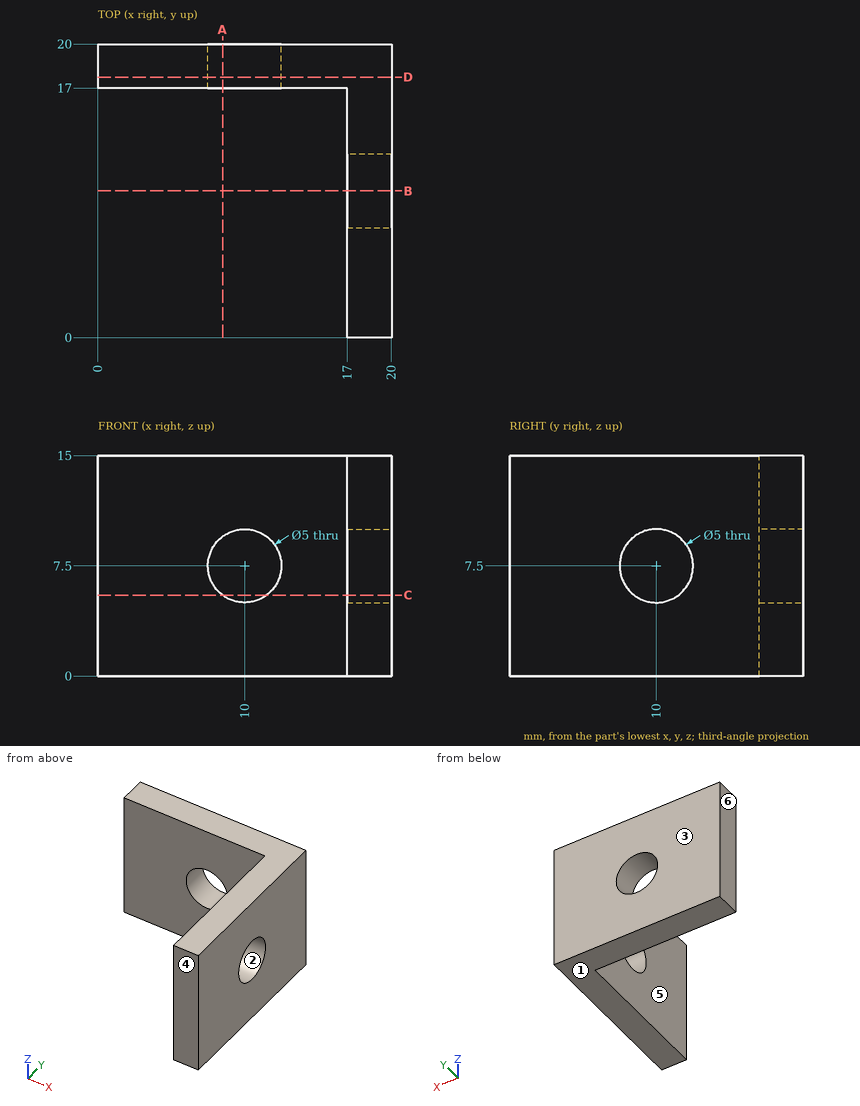
Could you check a few things on this drawing? It's one solid part, dimensions in mm from its lowest x, y, z. A direction names the side the tool comes from. Round coordinates to 2 decimals unless told otherwise and drop trailing zeros. Order: outer loops, then holes, each group sorted by start corner. A loop starts at its lowest first (then second) coordinate and runs counter-clockwise, first axis right, second up. Notation, with made-up numbers: M 76.25,36 L 110.25,36 A36 cw 110.25,75 Z; hole C 36.25,47.5 d3. An arc over 180 degrees is marked long. One line per question, with ' | ' between items. Start each with the question number.
(1) Suppose I cut it at A-A on x = 8.5. List the corners of the cut face in (y, z) for me, then the cut area to 3 significant figures.
(2) Suppose I cut it at B-B on y = 10. List the corners of the cut face in (x, z) for me, then the cut area to 3 significant figures.
(3) Suppose I cut it at C-C on z = 5.5. List the corners of the cut face in (x, y) for me, then the cut area to 3 significant figures.
(4) For P1, Ø5, axis at x = 8.5, y = 14, coming from the +Z side; P2, Ø7.5, axis at x = 11, z = 5, coming from the -Y side; P3, Ø6.5, axis at y = 10, z = 7.5, coming from the -X side, each with a flat end and sliding along its axis, tell me the tip position at first contact or that it passes through.
(5) Thinking about a two-plate mould opening in Y: for the marked faces 1, 2, 3 and 4, which applies, +Y half, -Y half, draft (parallel to the pull), parting line (faces both ways), or undercut?
(6) Suppose I cut it at D-D on y = 17.75. List the corners of the cut face in (x, z) for me.
(7) Please list where these lines run through material, in increasing order: line 1 along X through (y, z) = (17.95, 7.5); line 2 along Z through (x, y) = (19, 10); line 3 along X through (y, z) = (2.5, 6.75).
(8) For the marked faces 5 and 6, which set-ups out of +Z, -Z, +X, -X, +Y, -Y let a thin tool reach every point of the face, with its end or its side?
Geometry results:
1) outline: M 17,0 L 20,0 L 20,5.5 L 17,5.5 Z; M 17,9.5 L 20,9.5 L 20,15 L 17,15 Z | area: 33.0 mm²
2) outline: M 17,0 L 20,0 L 20,5 L 17,5 Z; M 17,10 L 20,10 L 20,15 L 17,15 Z | area: 30.0 mm²
3) outline: M 0,17 L 8.5,17 L 8.5,20 L 0,20 Z; M 11.5,17 L 17,17 L 17,11.5 L 20,11.5 L 20,20 L 11.5,20 Z; M 17,0 L 20,0 L 20,8.5 L 17,8.5 Z | area: 93.0 mm²
4) P1: through | P2: y = 17 | P3: x = 17
5) face 1: draft | face 2: undercut | face 3: +Y half | face 4: -Y half
6) outline: M 0,0 L 20,0 L 20,15 L 0,15 Z; hole C 10,7.5 d5
7) line 1: 0 to 7.5, 12.5 to 20 | line 2: 0 to 5, 10 to 15 | line 3: 17 to 20
8) face 5: +Z, -Z, -X, -Y | face 6: +Z, -Z, -X, +Y, -Y
